from build123d import *

# Parameters (mm, degrees)
BOSS_EXTRUDE1_DEPTH = 3.175
SKETCH2_R           = 1.2192
CUT_EXTRUDE1_DEPTH  = 4.175


with BuildPart() as part:
    # Sketch1 → Boss-Extrude1 (new body)
    with BuildSketch(Plane.XY):
        Polygon((-38.735, 6.35), (-41.91, 6.35), (-41.91, -6.35), (-38.735, -6.35), (-38.735, -28.575), (-6.35, -28.575), (-6.35, -31.75), (6.35, -31.75), (6.35, -28.575), (38.735, -28.575), (38.735, -6.35), (41.91, -6.35), (41.91, 6.35), (38.735, 6.35), (38.735, 28.575), (6.35, 28.575), (6.35, 31.75), (-6.35, 31.75), (-6.35, 28.575), (-38.735, 28.575), align=None)
    extrude(amount=BOSS_EXTRUDE1_DEPTH)

    # Sketch2 → Cut-Extrude1 (cut, through all)
    with BuildSketch(Plane.XY.offset(3.175)):
        with Locations((-22.86, 15.875)):
            Circle(SKETCH2_R)
        with Locations((22.86, 15.875)):
            Circle(SKETCH2_R)
        with Locations((22.86, -1.905)):
            Circle(SKETCH2_R)
        with Locations((-22.86, -1.905)):
            Circle(SKETCH2_R)
    extrude(amount=-CUT_EXTRUDE1_DEPTH, mode=Mode.SUBTRACT)


solid = part.part
Model file for the job. Use its own axes, mm. A direction names the side the tool comes from. Coordinates: 2 decimals unless noted, no trailing zeros. Order: outer loops, then holes, each group sorted by start corner. A loop starts at its lowest first (then second) coordinate and runs counter-clockwise, first axis right, second up. Notation, with made-up numbers: (-22, 56.5) -> (-2, 56.5) arc R21 cw to (-2, 87.5) -> close; hole circle Ø5 at (-37.5, 15.5). An arc over 180 degrees is marked (long way). Return JSON: item names as keys, results as strings. Group by question number.
Item 1: Wall check: line 1 along Y through (x, z) = (-22.86, 1.8) (3 decimals); line 2 along X through (y, z) = (27, 2.55) (3 decimals); line 3 along Y through (x, z) = (-31.5, 0.4) (3 decimals). Give the ranges that are in metal, low to high. Write a range as [from, to].
Item 2: Pull direction X, two halves, no side cores. Call faces 1 (the flat face through (41.91, 0, 2)), 2 (the cylindrical face through (21.892, -2.647, 1.61)), 3 (the flat face through (40, 6.35, 2)), 4 (the cylindrical face through (-22.3, 14.79, 1.61)): pulls with the +X half, pulls with the -X half, needs draft (parallel to the pull), parting line crosses it, or undercut.
Item 3: Saw through at C-C on x = 16. Write the cut outline in (y, z) (3 decimals), then the cut area to 3 significant figures.
Item 4: Saw through at A-A on x = -22.86. Write the cut outline in (y, z) (3 decimals).
Item 5: Saw through at D-D on y = 23. Write the cut outline in (x, z) (3 decimals).
Item 6: Flat gauge pins, fed straight in: P1, Ø1.5, axis at x = -22.86, y = 15.875, coming from the +Z side; P2, Ø1, axis at y = 13.5, z = 2, coming from the -X side (3 decimals); P3, Ø1.6, axis at y = -30.5, z = 1, coming from the +X side; P4, Ø1.6, axis at x = -40.5, z = 1, coming from the -Y side. Where does each tip first touch, or does it go through?
Item 7: Tool access for faces 5 (the flat face through (38.735, 17, 2)), 6 (the flat face through (-1, 0, 0)), 7 (the flat face through (40, -6.35, 2)), 8 (the flat face through (-22, 28.575, 2)), 9 (the flat face through (-38.735, -17, 2)): list every direction of +Z, -Z, +X, -X, +Y, -Y with a clear straight run to the whole face (end or side of a thin tool).
Item 8: Saw through at B-B on z = 0.5. Write the cut outline in (x, y) (3 decimals), then the cut area to 3 significant figures.
Values found:
{
 "1": {"line 1": "y = [-28.575, -3.124], [-0.686, 14.656], [17.094, 28.575]", "line 2": "x = [-38.735, 38.735]", "line 3": "y = [-28.575, 28.575]"},
 "2": {"face 1": "pulls with the +X half", "face 2": "undercut", "face 3": "needs draft", "face 4": "undercut"},
 "3": {"outline": "(-28.575, 0) -> (28.575, 0) -> (28.575, 3.175) -> (-28.575, 3.175) -> close", "area": "181 mm2"},
 "4": {"outline": "(-28.575, 0) -> (-3.124, 0) -> (-3.124, 3.175) -> (-28.575, 3.175) -> close; (-0.686, 0) -> (14.656, 0) -> (14.656, 3.175) -> (-0.686, 3.175) -> close; (17.094, 0) -> (28.575, 0) -> (28.575, 3.175) -> (17.094, 3.175) -> close"},
 "5": {"outline": "(-38.735, 0) -> (38.735, 0) -> (38.735, 3.175) -> (-38.735, 3.175) -> close"},
 "6": {"P1": "passes through", "P2": "stops at x = -38.735", "P3": "stops at x = 6.35", "P4": "stops at y = -6.35"},
 "7": {"face 5": "+Z, -Z, +X, +Y", "face 6": "-Z, +X, -X, +Y, -Y", "face 7": "+Z, -Z, +X, -Y", "face 8": "+Z, -Z, -X, +Y", "face 9": "+Z, -Z, -X, -Y"},
 "8": {"outline": "(-41.91, -6.35) -> (-38.735, -6.35) -> (-38.735, -28.575) -> (-6.35, -28.575) -> (-6.35, -31.75) -> (6.35, -31.75) -> (6.35, -28.575) -> (38.735, -28.575) -> (38.735, -6.35) -> (41.91, -6.35) -> (41.91, 6.35) -> (38.735, 6.35) -> (38.735, 28.575) -> (6.35, 28.575) -> (6.35, 31.75) -> (-6.35, 31.75) -> (-6.35, 28.575) -> (-38.735, 28.575) -> (-38.735, 6.35) -> (-41.91, 6.35) -> close; hole circle Ø2.438 at (-22.86, -1.905); hole circle Ø2.438 at (-22.86, 15.875); hole circle Ø2.438 at (22.86, -1.905); hole circle Ø2.438 at (22.86, 15.875)", "area": "4,570 mm2"}
}
